Build history of the part. All positions in model axes, mm. Coordinates: 2 decimals unless noted, no trailing zeros. Write each loop counter-clockwise with the first axis right and the second up, starting at its lowest first coordinate (ties: lowest second). Pieces come first, ordered by that corner, then holes.
from build123d import *

# Parameters (mm, degrees)
F0_W             = 254
F0_H             = 355.6
F1_DEPTH         = 6.35
F2_W             = 50.8
F2_H             = 6.35
F3_DEPTH         = 6.351
F3_COPIES2_COUNT = 2
F3_COPIES3_COUNT = 2
F3_COPIES3_ANGLE = 90
F3_COPIES4_COUNT = 2
F3_COPIES4_ANGLE = 90
F4_W             = 6.35
F4_H             = 50.8
F5_DEPTH         = 25.4
F6_W             = 76.2
F6_H             = 6.35
F7_DEPTH         = 25.4
F9_DEPTH         = 25.4


# Not quite as in the source:
# - a pattern or mirror of a feature is missing from the dataset's text; its kind, count and spacing are read off the source's solid


with BuildPart() as f1:
    # F0 (on Top) → F1 (new body)
    with BuildSketch(Plane.XY):
        Rectangle(F0_W, F0_H)
    extrude(amount=F1_DEPTH)

    # F2 (on face) → F3 (cut, through all)
    with BuildSketch(Plane.XY.offset(6.35)):
        with Locations((-76.2, 174.625)):
            Rectangle(F2_W, F2_H)
    f3 = extrude(amount=-F3_DEPTH, mode=Mode.SUBTRACT)

    # F3_copies: F3 across plane
    add(f3.mirror(Plane(origin=(0, 0, 0), x_dir=(0, 0, -1), z_dir=(0, -1, 0))), mode=Mode.SUBTRACT)

    # F3_copies1: F3 across plane
    add(f3.mirror(Plane(origin=(0, 0, 0), x_dir=(0, 0, 1), z_dir=(1, 0, 0))), mode=Mode.SUBTRACT)

    # F3_copies2: F3 ×2 about axis
    f3_copies2_axis = Axis((0, 0, 0), (0, 0, 1))
    for i in range(1, F3_COPIES2_COUNT):
        add(f3.rotate(f3_copies2_axis, i * 360 / F3_COPIES2_COUNT), mode=Mode.SUBTRACT)

    # F3_copies3: F3 ×2 about axis
    f3_copies3_axis = Axis((50.8, 0, 0), (0, 0, 1))
    for i in range(1, F3_COPIES3_COUNT):
        add(f3.rotate(f3_copies3_axis, i * F3_COPIES3_ANGLE / (F3_COPIES3_COUNT - 1)), mode=Mode.SUBTRACT)

    # F3_copies4: F3 ×2 about axis
    f3_copies4_axis = Axis((-76.2, 127, 0), (0, 0, 1))
    for i in range(1, F3_COPIES4_COUNT):
        add(f3.rotate(f3_copies4_axis, i * F3_COPIES4_ANGLE / (F3_COPIES4_COUNT - 1)), mode=Mode.SUBTRACT)

    # F4 (on face) → F5 (cut)
    with BuildSketch(Plane.XY.offset(6.35)):
        with Locations((123.825, 127)):
            Rectangle(F4_W, F4_H)
        with Locations((123.825, -127)):
            Rectangle(F4_W, F4_H)
    extrude(amount=-F5_DEPTH, mode=Mode.SUBTRACT)

    # F6 (on face) → F7 (cut)
    with BuildSketch(Plane.XY.offset(6.35)):
        with Locations((0, -85.725)):
            Rectangle(F6_W, F6_H)
    extrude(amount=-F7_DEPTH, mode=Mode.SUBTRACT)

    # F8 (on face) → F9 (cut)
    with BuildSketch(Plane.XY.offset(6.35)):
        with BuildLine():
            Line((0, 98.5919060208), (19.05, 130.4880061596))
            ThreePointArc((19.05, 130.4880061596), (0, 149.8517760723), (-19.05, 130.4880061596))
            Line((-19.05, 130.4880061596), (0, 98.5919060208))
        make_face()
    extrude(amount=-F9_DEPTH, mode=Mode.SUBTRACT)


solid = f1.part
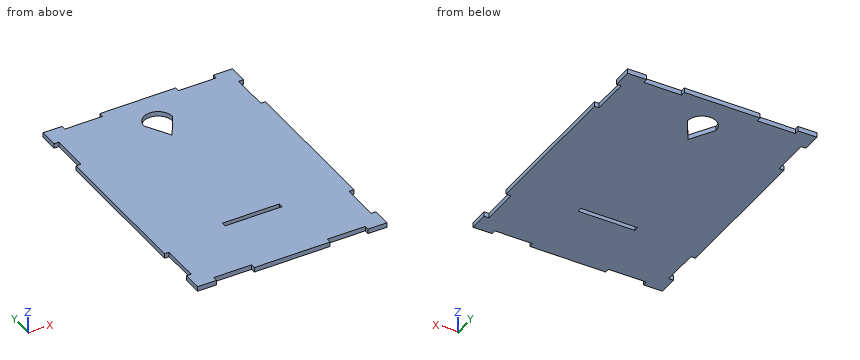
(1) Slice it at A-A, the plane y = 114. List the corners of the cut face in (x, z).
(2) Slice it at B-B, the plane x = 88. List the corners of the cut face in (y, z).
(3) Probe L1, parallel to Y at x = -25, z = 3.25; L2, parallel to Y at x = -11.5, z = 1.75; L3, parallel to Y at x = 8, z = 2. List the from-to ranges inside material, lowest first.
(4) Flat gauge pins, fed straight in: P1, Ø2, axis at x = 91, z = 1.5, coming from the -Y side; P2, Ø3, axis at x = 74.5, z = 4.5, coming from the +Y side; P3, Ø3, axis at x = 85, z = 3.5, coming from the -Y side. Where does each tip first touch, or does it go through?
Results:
1. outline: (-120.65, 0) - (-9.2, 0) - (-9.2, 6.35) - (-120.65, 6.35) - close; (9.2, 0) - (120.65, 0) - (120.65, 6.35) - (9.2, 6.35) - close
2. outline: (-171.45, 0) - (171.45, 0) - (171.45, 6.35) - (-171.45, 6.35) - close
3. L1: y = -177.8 to -88.9, -82.55 to 177.8
3. L2: y = -177.8 to -88.9, -82.55 to 117.85, 145.99 to 177.8
3. L3: y = -177.8 to -88.9, -82.55 to 111.99, 148.09 to 177.8
4. P1: stops at y = -171.45
4. P2: stops at y = 171.45
4. P3: stops at y = -171.45
